The model under review builds one solid part; all positions refer to its coordinate system, in mm. Face numbers are marked on the shaded views. A direction names the side the tool comes from. Coordinates: 2 decimals unless noted, no trailing zeros. Order: outer loops, then holes, each group sorted by start corner. A loop starts at its lowest first (then second) coordinate and runs counter-clockwise, first axis right, second up.
```python
from build123d import *

# Parameters (mm, degrees)
SKETCH1_W           = 180
SKETCH1_H           = 60
BOSS_EXTRUDE1_DEPTH = 10
CUT_EXTRUDE1_DEPTH  = 10
SKETCH3_W           = 10
SKETCH3_H           = 60
BOSS_EXTRUDE2_DEPTH = 40
SKETCH4_W           = 10
SKETCH4_H           = 40
BOSS_EXTRUDE3_DEPTH = 20
CUT_EXTRUDE2_DEPTH  = 20
SKETCH6_W           = 10
SKETCH6_H           = 40
BOSS_EXTRUDE4_DEPTH = 20
CUT_EXTRUDE3_DEPTH  = 20
BOSS_EXTRUDE5_DEPTH = 20
SKETCH10_R          = 10
CUT_EXTRUDE4_DEPTH  = 20
SKETCH11_W          = 50
SKETCH11_H          = 25
CUT_EXTRUDE5_DEPTH  = 20
SKETCH12_W          = 60
SKETCH12_H          = 20
BOSS_EXTRUDE6_DEPTH = 10


with BuildPart() as part:
    # Sketch1 → Boss-Extrude1 (new body)
    with BuildSketch(Plane(origin=(0, 0, 0), x_dir=(1, 0, 0), z_dir=(0, 1, 0))):
        with Locations((90, 30)):
            Rectangle(SKETCH1_W, SKETCH1_H)
    extrude(amount=BOSS_EXTRUDE1_DEPTH)

    # Sketch2 → Cut-Extrude1 (cut)
    with BuildSketch(Plane(origin=(0, 10, 0), x_dir=(1, 0, 0), z_dir=(0, 1, 0))):
        with BuildLine():
            Line((0, 60), (0, 40))
            ThreePointArc((0, 40), (10.963763172, 54.494897428), (28.284271247, 60))
            Line((28.284271247, 60), (0, 60))
        make_face()
        with BuildLine():
            Line((10, 40), (0, 40))
            Line((0, 40), (0, 20))
            Line((0, 20), (10, 20))
            ThreePointArc((10, 20), (20, 30), (10, 40))
        make_face()
        with BuildLine():
            ThreePointArc((28.284271247, 0), (10.963763172, 5.505102572), (0, 20))
            Line((0, 20), (0, 0))
            Line((0, 0), (28.284271247, 0))
        make_face()
        with BuildLine():
            ThreePointArc((180, 20), (169.036236828, 5.505102572), (151.715728753, 0))
            Line((151.715728753, 0), (180, 0))
            Line((180, 0), (180, 20))
        make_face()
        with BuildLine():
            Line((180, 20), (180, 40))
            Line((180, 40), (170, 40))
            ThreePointArc((170, 40), (160, 30), (170, 20))
            Line((170, 20), (180, 20))
        make_face()
        with BuildLine():
            Line((180, 60), (151.715728753, 60))
            ThreePointArc((151.715728753, 60), (169.036236828, 54.494897428), (180, 40))
            Line((180, 40), (180, 60))
        make_face()
    extrude(amount=-CUT_EXTRUDE1_DEPTH, mode=Mode.SUBTRACT)

    # Sketch3 → Boss-Extrude2 (add)
    with BuildSketch(Plane(origin=(0, 0, 0), x_dir=(-1, 0, 0), z_dir=(0, -1, 0))):
        with Locations((-55, 30)):
            Rectangle(SKETCH3_W, SKETCH3_H)
        with Locations((-125, 30)):
            Rectangle(SKETCH3_W, SKETCH3_H)
    extrude(amount=BOSS_EXTRUDE2_DEPTH)

    # Sketch4 → Boss-Extrude3 (add)
    with BuildSketch(Plane.ZY.offset(-50)):
        with Locations((-30, -20)):
            Rectangle(SKETCH4_W, SKETCH4_H)
    extrude(amount=BOSS_EXTRUDE3_DEPTH)

    # Sketch5 → Cut-Extrude2 (cut)
    with BuildSketch(Plane.XY.offset(-25)):
        Polygon((30, 0), (50, -40), (30, -40), align=None)
    extrude(amount=-CUT_EXTRUDE2_DEPTH, mode=Mode.SUBTRACT)

    # Sketch6 → Boss-Extrude4 (add)
    with BuildSketch(Plane(origin=(130, 0, 0), x_dir=(0, 0, -1), z_dir=(1, 0, 0))):
        with Locations((30, -20)):
            Rectangle(SKETCH6_W, SKETCH6_H)
    extrude(amount=BOSS_EXTRUDE4_DEPTH)

    # Sketch7 → Cut-Extrude3 (cut)
    with BuildSketch(Plane.XY.offset(-25)):
        Polygon((130, -40), (150, 0), (150, -40), align=None)
    extrude(amount=-CUT_EXTRUDE3_DEPTH, mode=Mode.SUBTRACT)

    # Sketch9 → Boss-Extrude5 (add)
    with BuildSketch(Plane.XZ.offset(40)):
        with BuildLine():
            Line((60, 0), (60, -60))
            ThreePointArc((60, -60), (67.071067812, -62.928932188), (70, -70))
            ThreePointArc((70, -70), (90, -90), (110, -70))
            ThreePointArc((110, -70), (112.928932188, -62.928932188), (120, -60))
            Line((120, -60), (120, 0))
            ThreePointArc((120, 0), (112.928932188, 2.928932188), (110, 10))
            ThreePointArc((110, 10), (90, 30), (70, 10))
            ThreePointArc((70, 10), (67.071067812, 2.928932188), (60, 0))
        make_face()
    extrude(amount=-BOSS_EXTRUDE5_DEPTH)

    # Sketch10 → Cut-Extrude4 (cut)
    with BuildSketch(Plane(origin=(0, -20, 0), x_dir=(1, 0, 0), z_dir=(0, 1, 0))):
        with Locations((90, 70)):
            Circle(SKETCH10_R)
        with Locations((90, -10)):
            Circle(SKETCH10_R)
    extrude(amount=-CUT_EXTRUDE4_DEPTH, mode=Mode.SUBTRACT)

    # Sketch11 → Cut-Extrude5 (cut)
    with BuildSketch(Plane(origin=(0, 10, 0), x_dir=(1, 0, 0), z_dir=(0, 1, 0))):
        with Locations((85, 47.5)):
            Rectangle(SKETCH11_W, SKETCH11_H)
        with Locations((85, 12.5)):
            Rectangle(SKETCH11_W, SKETCH11_H)
    extrude(amount=-CUT_EXTRUDE5_DEPTH, mode=Mode.SUBTRACT)

    # Sketch12 → Boss-Extrude6 (add)
    with BuildSketch(Plane.XY.offset(-25)):
        with Locations((90, -10)):
            Rectangle(SKETCH12_W, SKETCH12_H)
    extrude(amount=-BOSS_EXTRUDE6_DEPTH)


solid = part.part
```
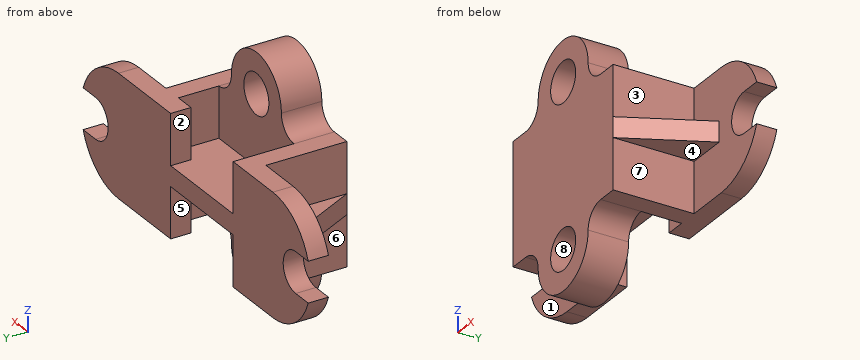
(1) We need section A-A, the plane z = -64. Write out the cut boundary in (x, y).
A:
outline: (68, -40) - (82, -40) - (82, -20) - (68, -20) - close; (98, -40) - (112, -40) - (112, -20) - (98, -20) - close
(2) We need section B-B, the plane x = 90. Write out the cut boundary in (y, z).
A:
outline: (-40, -90) - (-20, -90) - (-20, -80) - (-40, -80) - close; (-40, -60) - (-20, -60) - (-20, -35) - (10, -35) - (10, -25) - (-20, -25) - (-20, 0) - (-40, 0) - close; (-40, 20) - (-20, 20) - (-20, 30) - (-40, 30) - close
(3) Machinability: for the marked faces 1, 2, 3, 4 and 5, which of the approach directions +Z, -Z, +X, -X, +Y, -Y give a long, thin tool a straight path to every point of the face, cutting with its end or side? Answer none if there is none.
A:
face 1: -X, -Y
face 2: +Z, +Y
face 3: +Z, +X, -Y
face 4: -Z, +X, -Y
face 5: -Z, +Y
(4) Wall thickness on probe 1 along Z at (x, y) = (90, -32.75); probe 2 along X at (y, z) = (-27, 10); probe 3 along Z at (x, y) = (43.5, -1): over which ranges is each line inside the solid? List them lowest first.
A:
probe 1: z = -90 to -80, -60 to 0, 20 to 30
probe 2: x = 70 to 80, 100 to 110
probe 3: z = -35 to -25
(5) Draft analysis for pull direction X (two halves, no side actions). For the marked faces 6, 7 and 8, state which applies: released by +X, released by -X, zero draft, split by the parting line, or undercut.
A:
face 6: released by -X
face 7: released by +X
face 8: undercut
(6) For pin 1 Ø7.5 at (y, z) = (-16.5, -51) entering from +X; pin 2 Ø1.5 at (x, y) = (78.5, -14) entering from +Z; pin 3 Ø24 at (x, y) = (103, -2) entering from -Z, all flat-tipped, find the tip position at first contact; note any pin that passes through.
A:
pin 1: stops at x = 130
pin 2: stops at z = -25
pin 3: stops at z = -60
(7) We need section C-C, the plane y = -3. Write out the cut boundary in (x, z).
A:
outline: (31.5, -35) - (50, -35) - (50, -60) - (60, -60) - (60, -35) - (120, -35) - (120, -60) - (130, -60) - (130, -35) - (148.5, -35) - (148.5, -25) - (130, -25) - (130, 0) - (120, 0) - (120, -25) - (60, -25) - (60, 0) - (50, 0) - (50, -25) - (31.5, -25) - close
(8) We need section D-D, the plane z = -30. Write out the cut boundary in (x, y), and give its area (3 significant figures).
A:
outline: (20, 0) - (30, 0) - (50, -40) - (130, -40) - (150, 0) - (160, 0) - (160, 10) - (20, 10) - close
area: 5,400 mm2
